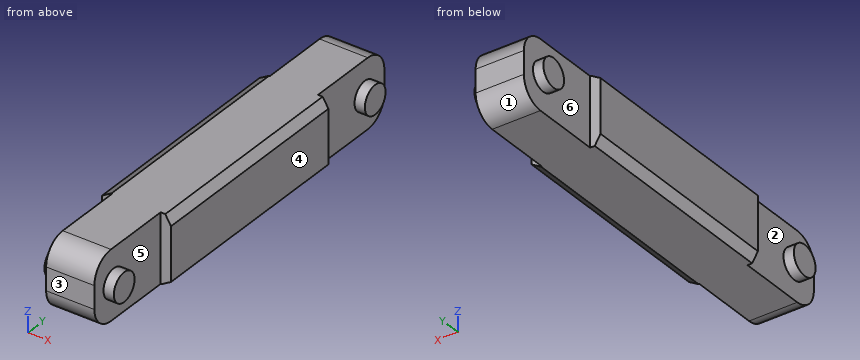
from build123d import *

# Parameters (mm, degrees)
SKETCH1_W             = 120
SKETCH1_H             = 120
BOSS_EXTRUDE1_DEPTH   = 700
SKETCH2_W             = 18
SKETCH2_H             = 120
CUT_EXTRUDE1_DEPTH    = 160
SKETCH3_R             = 26.228524845
BOSS_EXTRUDE2_DEPTH   = 18
SKETCH4_R             = 25
BOSS_EXTRUDE3_DEPTH   = 18
FILLET1_R             = 40
SKETCH5_W             = 18
SKETCH5_H             = 120
CUT_EXTRUDE2_DEPTH    = 160
SKETCH6_R             = 25
BOSS_EXTRUDE5_DEPTH   = 18
SKETCH7_R             = 25
BOSS_EXTRUDE6_DEPTH   = 18
FILLET2_R             = 40
CHAMFER1_SIZE         = 10
CHAMFER1_SIZE2        = 16.642794824
CHAMFER1_PART_2_SIZE  = 10
CHAMFER1_PART_2_SIZE2 = 16.642794824
CHAMFER1_PART_3_SIZE  = 10
CHAMFER1_PART_3_SIZE2 = 16.642794824
CHAMFER1_PART_4_SIZE  = 10
CHAMFER1_PART_4_SIZE2 = 16.642794824


with BuildPart() as part:
    # Sketch1 → Boss-Extrude1 (new body)
    with BuildSketch(Plane(origin=(0, 0, 0), x_dir=(1, 0, 0), z_dir=(0, 1, 0))):
        Rectangle(SKETCH1_W, SKETCH1_H)
    extrude(amount=BOSS_EXTRUDE1_DEPTH)

    # Sketch2 → Cut-Extrude1 (cut)
    with BuildSketch(Plane.XZ):
        with Locations((-51, 0)):
            Rectangle(SKETCH2_W, SKETCH2_H)
        with Locations((51, 0)):
            Rectangle(SKETCH2_W, SKETCH2_H)
    extrude(amount=-CUT_EXTRUDE1_DEPTH, mode=Mode.SUBTRACT)

    # Sketch3 → Boss-Extrude2 (add)
    with BuildSketch(Plane.ZY.offset(42)):
        with Locations((0, 47.02)):
            Circle(SKETCH3_R)
    extrude(amount=BOSS_EXTRUDE2_DEPTH)

    # Sketch4 → Boss-Extrude3 (add)
    with BuildSketch(Plane(origin=(42, 0, 0), x_dir=(0, 0, -1), z_dir=(1, 0, 0))):
        with Locations((0, 47.02)):
            Circle(SKETCH4_R)
    extrude(amount=BOSS_EXTRUDE3_DEPTH)

    # Fillet1
    fillet1_edges = [part.edges().sort_by_distance(p)[0] for p in [
        (0, 0, 60),
        (0, 0, -60),
    ]]
    fillet(fillet1_edges, radius=FILLET1_R)

    # Sketch5 → Cut-Extrude2 (cut)
    with BuildSketch(Plane(origin=(0, 700, 0), x_dir=(1, 0, 0), z_dir=(0, 1, 0))):
        with Locations((-51, 0)):
            Rectangle(SKETCH5_W, SKETCH5_H)
        with Locations((51, 0)):
            Rectangle(SKETCH5_W, SKETCH5_H)
    extrude(amount=-CUT_EXTRUDE2_DEPTH, mode=Mode.SUBTRACT)

    # Sketch6 → Boss-Extrude5 (add)
    with BuildSketch(Plane.ZY.offset(42)):
        with Locations((0, 652.98)):
            Circle(SKETCH6_R)
    extrude(amount=BOSS_EXTRUDE5_DEPTH)

    # Sketch7 → Boss-Extrude6 (add)
    with BuildSketch(Plane(origin=(42, 0, 0), x_dir=(0, 0, -1), z_dir=(1, 0, 0))):
        with Locations((0, 652.98)):
            Circle(SKETCH7_R)
    extrude(amount=BOSS_EXTRUDE6_DEPTH)

    # Fillet2
    fillet2_edges = [part.edges().sort_by_distance(p)[0] for p in [
        (0, 700, -60),
        (0, 700, 60),
    ]]
    fillet(fillet2_edges, radius=FILLET2_R)

    # Chamfer1
    chamfer1_edges = [part.edges().sort_by_distance(p)[0] for p in [
        (60, 350, 60),
    ]]
    chamfer1_side = [part.faces().sort_by_distance(p)[0] for p in [
        (0, 350, 60),
    ]]
    chamfer(chamfer1_edges, length=CHAMFER1_SIZE, length2=CHAMFER1_SIZE2, reference=chamfer1_side[0])

    # Chamfer1 part 2
    chamfer1_part_2_edges = [part.edges().sort_by_distance(p)[0] for p in [
        (-60, 350, 60),
    ]]
    chamfer1_part_2_side = [part.faces().sort_by_distance(p)[0] for p in [
        (-60, 350, 0),
    ]]
    chamfer(chamfer1_part_2_edges, length=CHAMFER1_PART_2_SIZE, length2=CHAMFER1_PART_2_SIZE2, reference=chamfer1_part_2_side[0])

    # Chamfer1 part 3
    chamfer1_part_3_edges = [part.edges().sort_by_distance(p)[0] for p in [
        (-60, 350, -60),
    ]]
    chamfer1_part_3_side = [part.faces().sort_by_distance(p)[0] for p in [
        (0, 350, -60),
    ]]
    chamfer(chamfer1_part_3_edges, length=CHAMFER1_PART_3_SIZE, length2=CHAMFER1_PART_3_SIZE2, reference=chamfer1_part_3_side[0])

    # Chamfer1 part 4
    chamfer1_part_4_edges = [part.edges().sort_by_distance(p)[0] for p in [
        (60, 350, -60),
    ]]
    chamfer1_part_4_side = [part.faces().sort_by_distance(p)[0] for p in [
        (60, 350, 0),
    ]]
    chamfer(chamfer1_part_4_edges, length=CHAMFER1_PART_4_SIZE, length2=CHAMFER1_PART_4_SIZE2, reference=chamfer1_part_4_side[0])


solid = part.part
Model file for the job. Use its own axes, mm. Face numbers are marked on the shaded views. A direction names the side the tool comes from. Round coordinates to 2 decimals unless told otherwise and drop trailing zeros. Order: outer loops, then holes, each group sorted by start corner. A loop starts at its lowest first (then second) coordinate and runs counter-clockwise, first axis right, second up.
(1) Band-saw the part on D-D (y = 652.98). List the corners of the cut face in (x, z), then the cut area to 3 significant figures.
(2) Band-saw the part on B-B (x = 18). List the corners of the cut face in (y, z).
(3) Band-saw the part on A-A (y = 353). List the corners of the cut face in (x, z), then the cut area to 3 significant figures.
(4) Band-saw the part on C-C (z = 0). List the corners of the cut face in (x, y), then the cut area to 3 significant figures.
(5) 3-axis set-ups, long thin cutter, end or side, ignore diameter. For the marked faces 4, 5 and 6: which of +Z, -Z, +X, -X, +Y, -Y reach the whole face in a straight line?
(6) Pin check, flat tips, straight feed: pin 1 (5 mm diameter, centred on x = 29, z = 47.5, fed in from +Y) (3 decimals); pin 2 (5.5 mm diameter, centred on x = 53.5, z = -20.5, fed in from -Y); pin 3 (5.5 mm diameter, centred on x = -51.5, z = 2.5, fed in from -Y); pin 4 (20 mm diameter, centred on x = -49.5, z = -4.5, fed in from +Y). Stop position of each tip, or through.
(7) Drill centre lines: line 1 (Y direction, x = -51.5, z = 5); line 2 (X direction, y = 114, z = 25.5); line 3 (Y direction, x = 53, z = -42.5). Where is each one in solid material? Low to high.
(8) Pull direction Y, two halves, no side cores. Call the marked faces 1, 2 and 3: released by +Y, released by -Y, zero draft, split by the parting line, or undercut.
Verdict:
1. outline: (-60, -25) - (-42, -25) - (-42, -60) - (42, -60) - (42, -25) - (60, -25) - (60, 25) - (42, 25) - (42, 60) - (-42, 60) - (-42, 25) - (-60, 25) - close
1. area: 11,900 mm2
2. outline: (0, -20) arc R40 ccw to (40, -60) - (660, -60) arc R40 ccw to (700, -20) - (700, 20) arc R40 ccw to (660, 60) - (40, 60) arc R40 ccw to (0, 20) - close
3. outline: (-60, -43.36) - (-50, -60) - (43.36, -60) - (60, -50) - (60, 43.36) - (50, 60) - (-43.36, 60) - (-60, 50) - close
3. area: 14,100 mm2
4. outline: (-60, 20.79) - (-42, 20.79) - (-42, 0) - (42, 0) - (42, 22.02) - (60, 22.02) - (60, 72.02) - (42, 72.02) - (42, 160) - (60, 160) - (60, 540) - (42, 540) - (42, 627.98) - (60, 627.98) - (60, 677.98) - (42, 677.98) - (42, 700) - (-42, 700) - (-42, 677.98) - (-60, 677.98) - (-60, 627.98) - (-42, 627.98) - (-42, 540) - (-60, 540) - (-60, 160) - (-42, 160) - (-42, 73.25) - (-60, 73.25) - close
4. area: 76,100 mm2
5. face 4: +Z, -Z, +X, +Y, -Y
5. face 5: +X
5. face 6: -X
6. pin 1: stops at y = 691.225
6. pin 2: stops at y = 29.41
6. pin 3: stops at y = 20.79
6. pin 4: stops at y = 700
7. line 1: y = 21.27 to 72.77, 160 to 540, 628.49 to 677.47
7. line 2: x = -42 to 42
7. line 3: y = 160 to 540
8. face 1: released by +Y
8. face 2: undercut
8. face 3: released by -Y
